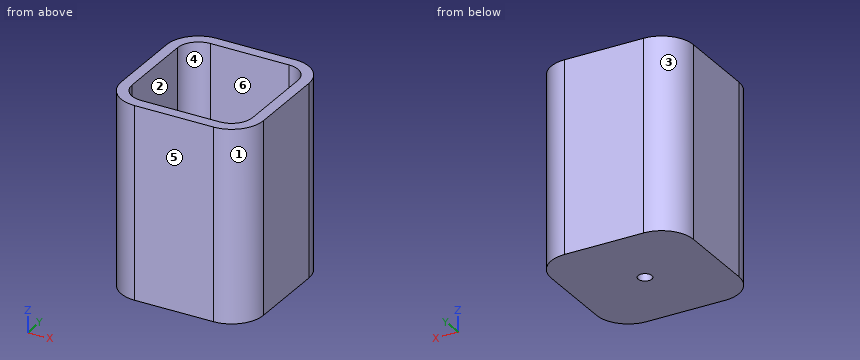
```python
from build123d import *

# Parameters (mm, degrees)
F1_DEPTH = 35
F2_DEPTH = 2
F3_D     = 2.5


with BuildPart() as f1:
    # F0 (on Top) → F1 (new body)
    with BuildSketch(Plane.XY):
        with BuildLine():
            Line((13, -7.19), (13, 7.19))
            ThreePointArc((13, 7.19), (11.29829, 11.29829), (7.19, 13))
            Line((7.19, 13), (-7.19, 13))
            ThreePointArc((-7.19, 13), (-11.29829, 11.29829), (-13, 7.19))
            Line((-13, 7.19), (-13, -7.19))
            ThreePointArc((-13, -7.19), (-11.29829, -11.29829), (-7.19, -13))
            Line((-7.19, -13), (7.19, -13))
            ThreePointArc((7.19, -13), (11.29829, -11.29829), (13, -7.19))
        make_face()
        with BuildLine():
            ThreePointArc((-11, 7.19), (-9.884077, 9.884077), (-7.19, 11))
            Line((-7.19, 11), (7.19, 11))
            ThreePointArc((7.19, 11), (9.884077, 9.884077), (11, 7.19))
            Line((11, 7.19), (11, -7.19))
            ThreePointArc((11, -7.19), (9.884077, -9.884077), (7.19, -11))
            Line((7.19, -11), (-7.19, -11))
            ThreePointArc((-7.19, -11), (-9.884077, -9.884077), (-11, -7.19))
            Line((-11, -7.19), (-11, 7.19))
        make_face(mode=Mode.SUBTRACT)
    extrude(amount=F1_DEPTH)

    # F0 (on Top) → F2 (join)
    with BuildSketch(Plane.XY):
        with BuildLine():
            Line((7.19, 11), (-7.19, 11))
            ThreePointArc((-7.19, 11), (-9.884077, 9.884077), (-11, 7.19))
            Line((-11, 7.19), (-11, -7.19))
            ThreePointArc((-11, -7.19), (-9.884077, -9.884077), (-7.19, -11))
            Line((-7.19, -11), (7.19, -11))
            ThreePointArc((7.19, -11), (9.884077, -9.884077), (11, -7.19))
            Line((11, -7.19), (11, 7.19))
            ThreePointArc((11, 7.19), (9.884077, 9.884077), (7.19, 11))
        make_face()
    extrude(amount=F2_DEPTH)

    # F3 (through all)
    with Locations(Plane(origin=(0, 0, 0), x_dir=(1, 0, 0), z_dir=(0, 0, -1))):
        with Locations((0, 0)):
            Hole(F3_D / 2)


solid = f1.part
```
Input: part model. Units: mm. Frame: model coordinates. Face numbers are marked on the shaded views. A direction names the side the tool comes from. Coordinates: 2 decimals unless noted, no trailing zeros. Loops run counter-clockwise (first coordinate to the right, second up) from the corner with the lowest first, then second, coordinate; pieces in that order, holes last. Notation, with made-up numbers: M 39,43 L 52,43 A25 cw 52,70 Z; hole C 50.25,59.5 d3. An arc over 180 degrees is marked long. Use a Markdown table: item, result. Add a question column.
1) Section B-B, the plane z = 15. Return the cut outline in (x, y), plus the area to 3 significant figures.
2) Draft query along X for the marked faces 3, 4, 5 and 6. Return one class per face: +X half, -X half, draft (parallel to the pull), parting line (faces both ways), or undercut.
3) Section D-D, the plane x = -4.25. Return the cut outline in (y, z).
4) Pin query (flat end, axial travel): P1, Ø2, axis at x = 0, y = 0, coming from the +Z side; P2, Ø1, axis at x = 8, z = 16, coming from the +Y side; P3, Ø1, axis at x = 8, z = 11.5, coming from the -Y side; P4, Ø2, axis at x = 5, y = 9, coming from the +Z side. Return the tip coordinate at first contact, or that it passes through.
5) Section A-A, the plane y = 0. Return the cut outline in (x, z), plus the area to 3 significant figures.
6) Set-up query: the marked faces 1 and 2. Return all of +Z, -Z, +X, -X, +Y, -Y with unobstructed straight access to the full face (end or side cutting, diameter ignored); none if empty.
7) Line query: L1, parallel to X at y = -5.5, z = 31; L2, parallel to Y at x = 0, z = 1.35. Output: solid intervals per line, ascending. Write a range as from..to.
Answer below:
| question | item | result |
|---|---|---|
| 1 | outline | M -13,-7.19 A5.81 ccw -7.19,-13 L 7.19,-13 A5.81 ccw 13,-7.19 L 13,7.19 A5.81 ccw 7.19,13 L -7.19,13 A5.81 ccw -13,7.19 Z; hole M -11,-7.19 A3.81 ccw -7.19,-11 L 7.19,-11 A3.81 ccw 11,-7.19 L 11,7.19 A3.81 ccw 7.19,11 L -7.19,11 A3.81 ccw -11,7.19 Z |
| 1 | area | 175 mm2 |
| 2 | face 3 | -X half |
| 2 | face 4 | undercut |
| 2 | face 5 | draft |
| 2 | face 6 | undercut |
| 3 | outline | M -13,0 L 13,0 L 13,35 L 11,35 L 11,2 L -11,2 L -11,35 L -13,35 Z |
| 4 | P1 | through |
| 4 | P2 | y = 12.99 |
| 4 | P3 | y = -12.99 |
| 4 | P4 | z = 2 |
| 5 | outline | M -13,0 L -1.25,0 L -1.25,2 L -11,2 L -11,35 L -13,35 Z; M 1.25,0 L 13,0 L 13,35 L 11,35 L 11,2 L 1.25,2 Z |
| 5 | area | 179 mm2 |
| 6 | face 1 | +Z, -Z, +X, -Y |
| 6 | face 2 | +Z |
| 7 | L1 | -13..-11, 11..13 |
| 7 | L2 | -13..-1.25, 1.25..13 |
